Autodesk Inventor part; units mm, degrees
ref_plane "YZ Plane" through (0, 0, 0) normal (1, 0, 0) x (0, 1, 0)
ref_plane "XZ Plane" through (0, 0, 0) normal (0, 1, 0) x (-1, 0, 0)
ref_plane "XY Plane" through (0, 0, 0) normal (0, 0, 1) x (1, 0, 0)
sketch "Sketch1" plane through (0, 0, 0) normal (0, 0, 1) x (1, 0, 0)
  line L0 (-122.5, 115) -> (122.5, 115)
  line L1 (122.5, 115) -> (122.5, -115)
  line L2 (122.5, -115) -> (-122.5, -115)
  line L3 (-122.5, -115) -> (-122.5, 115)
  point P0 (0, 0)
  dimension "d0" = 245
  dimension "d1" = 230
  dimension "d2" = 122.5
  dimension "d3" = 115
extrude "Extrusion1" add sketch "Sketch1" along normal blind 10
sketch "Sketch2" plane through (0, 0, 10) normal (0, 0, 1) x (1, 0, 0)
  circle A0 centre (0, 0) radius 4
  dimension "d6" = 8
extrude "Extrusion2" cut sketch "Sketch2" against normal up to next
properties part number "Base" material "ABS Plastic"
For this review, take the finished solid that the model builds, in its own axes (mm). Coordinates: 2 decimals unless noted, no trailing zeros. Loops run counter-clockwise (first coordinate to the right, second up) from the corner with the lowest first, then second, coordinate; pieces in that order, holes last. Notation, with made-up numbers: (-3, -4.75) - (6, -4.75) arc R37 ccw to (6, 33.25) - close; hole circle Ø6 at (62.25, 69.5). An arc over 180 degrees is marked (long way). Use a Markdown table: item, result. Add a question column.
Item 1: We need section B-B (x = 0). Give the boundary of the cut face in (y, z).
Item 2: We need section A-A (y = 0). Give the boundary of the cut face in (x, z), and give its area (3 significant figures).
Item 3: For line 1 (Y direction, x = 0, z = 4); line 2 (X direction, y = 1, z = 9.5); line 3 (Y direction, x = -3, z = 4.75), list the stretches that pass through material, from the lowest coordinate up.
Item 4: Insertion check: pin 1 Ø4 at (x, y) = (84.5, -47.5) entering from -Z. The pin has a flat end and moves straight along its axis. Give the tip position at first contact, or say it passes through.
Item 5: Mouldability with a two-part tool opening along Y and no side actions: class faces 1 (the face through (-122.5, -2, 5)), 2 (the face through (2, -115, 5)), 3 (the face through (-0.867, -3.905, 5.07)) as pulls with the +Y half, pulls with the -Y half, needs draft (parallel to the pull), parting line crosses it, or undercut.
Results list:
| question | item | result |
|---|---|---|
| 1 | outline | (-115, 0) - (-4, 0) - (-4, 10) - (-115, 10) - close; (4, 0) - (115, 0) - (115, 10) - (4, 10) - close |
| 2 | outline | (-122.5, 0) - (-4, 0) - (-4, 10) - (-122.5, 10) - close; (4, 0) - (122.5, 0) - (122.5, 10) - (4, 10) - close |
| 2 | area | 2,370 mm^2 |
| 3 | line 1 | y = -115 to -4, 4 to 115 |
| 3 | line 2 | x = -122.5 to -3.87, 3.87 to 122.5 |
| 3 | line 3 | y = -115 to -2.65, 2.65 to 115 |
| 4 | pin 1 | stops at z = 0 |
| 5 | face 1 | needs draft |
| 5 | face 2 | pulls with the -Y half |
| 5 | face 3 | undercut |
